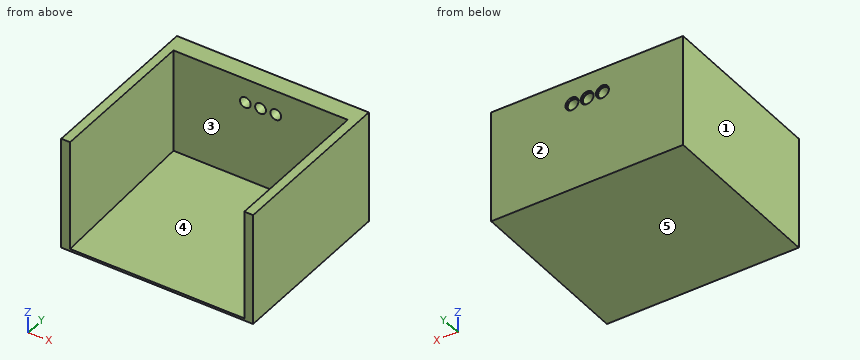
Autodesk Fusion 360 part; units mm, degrees
sketch "Sketch1" plane through (0, 0, 0) normal (0, 0, 1) x (1, 0, 0)
  line L0 (0, 0) -> (81, 0)
  line L1 (81, 0) -> (81, 71)
  line L2 (81, 71) -> (0, 71)
  line L3 (0, 71) -> (0, 0)
  dimension "d1" = 81
  dimension "d2" = 71
extrude "Extrude1" add sketch "Sketch1" along normal blind 1
sketch "Sketch2" plane through (0, 0, 0) normal (1, 0, 0) x (0, 1, 0)
sketch "Sketch3" plane through (0, 0, 1) normal (0, 0, 1) x (-1, 0, 0)
  line L0 (0, -71) -> (0, 0)
  line L1 (0, 0) -> (-81, 0)
  line L2 (-81, 0) -> (-81, -71)
  line L3 (-81, -71) -> (0, -71)
  line L4 (0, -71) -> (-1, -71)
  line L5 (-1, -71) -> (-1, 0)
  line L6 (-1, 0) -> (0, 0)
  line L7 (0, 0) -> (0, -71)
  line L8 (-81, -71) -> (-80, -71)
  line L9 (-80, -71) -> (-80, 0)
  line L10 (-80, 0) -> (-81, 0)
  line L11 (-81, 0) -> (-81, -71)
  line L12 (-1, -71) -> (-80, -71)
  line L13 (-80, -71) -> (-80, -70)
  line L14 (-80, -70) -> (-1, -70)
  line L15 (-1, -70) -> (-1, -71)
  dimension "d5" = 1
  dimension "d6" = 1
  dimension "d7" = 1
extrude "Extrude2" add sketch "Sketch3" along normal blind 50 contours L3 L5 L9 L12 L13 L14 L15
sketch "Sketch4" plane through (0, 0, 1) normal (0, 0, 1) x (-1, 0, 0)
  line L0 (-80, -71) -> (-80, -70)
  line L1 (-80, -70) -> (-1, -70)
  line L2 (-1, -70) -> (-1, -71)
  line L3 (-1, -71) -> (0, -71)
  line L4 (0, -71) -> (0, 0)
  line L5 (0, 0) -> (-81, 0)
  line L6 (-81, 0) -> (-81, -71)
  line L7 (-81, -71) -> (-80, -71)
  line L8 (0, 0) -> (-1, 0)
  line L9 (-1, 0) -> (-1, -71)
  line L10 (-1, -71) -> (0, -71)
  line L11 (0, -71) -> (0, 0)
  dimension "d10" = 1
  dimension "d11" = 71
extrude "Extrude3" add sketch "Sketch4" along normal blind 50 contours L2 L3 L4 L5 L8 L9 L10 L11
sketch "Sketch5" plane through (0, 0, 1) normal (0, 0, 1) x (-1, 0, 0)
  line L0 (-1, -70) -> (-1, 0)
  line L1 (-1, 0) -> (-81, 0)
  line L2 (-81, 0) -> (-81, -71)
  line L3 (-81, -71) -> (-80, -71)
  line L4 (-80, -71) -> (-80, -70)
  line L5 (-80, -70) -> (-1, -70)
  line L6 (-81, 0) -> (-80, 0)
  line L7 (-80, 0) -> (-80, -71)
  line L8 (-80, -71) -> (-81, -71)
  line L9 (-81, -71) -> (-81, 0)
  dimension "d14" = 71
extrude "Extrude4" add sketch "Sketch5" along normal blind 50 contours L1 L2 L3 L4 L6 L7 L8 L9
sketch "Sketch6" plane through (0, 70, 0) normal (0, -1, 0) x (1, 0, 0)
  line L0 (1, 1) -> (80, 1)
  line L1 (80, 1) -> (80, 51)
  line L2 (80, 51) -> (1, 51)
  line L3 (1, 51) -> (1, 1)
  line L4 (80, 1) -> (80, 4)
  line L5 (1, 4) -> (1, 1)
  dimension "d17" = 79
  dimension "d18" = 3
sketch "Sketch7" plane through (0, 70, 0) normal (0, -1, 0) x (1, 0, 0)
extrude "Extrude5" cut 1 faces at (27.3333, 46.6667, 1) along direction (0, 0, -1) blind 1
sketch "Sketch8" plane through (0, 0, 0) normal (0, 1, 0) x (1, 0, 0)
sketch "Sketch9" plane through (1, 0, 0) normal (1, 0, 0) x (0, 1, 0)
  line L0 (70, 0) -> (70, 51)
  line L1 (70, 51) -> (0, 51)
  line L2 (0, 51) -> (0, 0)
  line L3 (0, 0) -> (70, 0)
  line L4 (0, 0) -> (70, 0)
  line L5 (70, 0) -> (70, 1)
  line L6 (70, 1) -> (0, 1)
  line L7 (0, 1) -> (0, 0)
  dimension "d21" = 70
  dimension "d22" = 1
extrude "Extrude6" add sketch "Sketch9" along normal blind 79 contours L0 L2 L3 L4 L5 L6 L7
sketch "Sketch10" plane through (80, 0, 0) normal (-1, 0, 0) x (0, -1, 0)
  line L0 (-70, 1) -> (0, 1)
  line L1 (0, 1) -> (0, 51)
  line L2 (0, 51) -> (-70, 51)
  line L3 (-70, 51) -> (-70, 1)
  line L4 (-70, 1) -> (-70, 4)
  line L5 (-70, 4) -> (0, 1)
  line L6 (-70, 1) -> (-70, 4)
extrude "Extrude7" add sketch "Sketch10" along normal blind 79 contours L0 L3 L4 L5 L6
sketch "Sketch11" plane through (0, 0, 0) normal (0, 0, 1) x (1, 0, 0)
  line L0 (0, 0) -> (-3, 0)
  line L1 (-3, 0) -> (-3, 74)
  line L2 (-3, 74) -> (0, 74)
  line L3 (0, 74) -> (0, 0)
  dimension "d27" = 3
  dimension "d28" = 74
extrude "Extrude8" add sketch "Sketch11" along normal blind 51
sketch "Sketch12" plane through (0, 0, 0) normal (1, 0, 0) x (0, 1, 0)
  line L0 (71, 51) -> (71, 0)
  line L1 (71, 0) -> (74, 0)
  line L2 (74, 0) -> (74, 51)
  line L3 (74, 51) -> (71, 51)
  line L4 (74, 51) -> (71, 51)
  line L5 (71, 51) -> (71, 0)
  line L6 (71, 0) -> (74, 0)
  line L7 (74, 0) -> (74, 51)
extrude "Extrude9" add sketch "Sketch12" along normal blind 84
sketch "Sketch13" plane through (0, 71, 0) normal (0, -1, 0) x (1, 0, 0)
  line L0 (81, 51) -> (81, 0)
  line L1 (81, 0) -> (84, 0)
  line L2 (84, 0) -> (84, 51)
  line L3 (84, 51) -> (81, 51)
  line L4 (81, 51) -> (84, 51)
  line L5 (84, 51) -> (84, 0)
  line L6 (84, 0) -> (81, 0)
  line L7 (81, 0) -> (81, 51)
extrude "Extrude10" add sketch "Sketch13" along normal blind 71
sketch "Sketch14" plane through (0, 74, 0) normal (0, 1, 0) x (-1, 0, 0)
  line L0 (-84, 0) -> (3, 0)
  line L1 (3, 0) -> (3, 51)
  line L2 (3, 51) -> (-84, 51)
  line L3 (-84, 51) -> (-84, 0)
extrude "Extrude11" add sketch "Sketch14" along normal blind 4.3
sketch "Sketch15" plane through (0, 78.3, 0) normal (0, 1, 0) x (-1, 0, 0)
  line L0 (-84, 51) -> (-84, 0)
  line L1 (-84, 0) -> (3, 0)
  line L2 (3, 0) -> (3, 51)
  line L3 (3, 51) -> (-84, 51)
  line L4 (-79, 40) -> (-84, 40)
  circle A0 centre (-40.5, 40) radius 2.95
  dimension "d37" = 43.5
  dimension "d38" = 5.9
extrude "Extrude12" cut sketch "Sketch15" against normal blind 0.8 contours A0
sketch "Sketch16" plane through (0, 77.5, 0) normal (0, 1, 0) x (-1, 0, 0)
  circle A0 centre (-40.5, 40) radius 2.95
  circle A1 centre (-40.5, 40) radius 2.45
  dimension "d41" = 4.9
extrude "Extrude13" cut sketch "Sketch16" against normal blind 10 contours A1
sketch "Sketch17" plane through (0, 78.3, 0) normal (0, 1, 0) x (-1, 0, 0)
  circle A0 centre (-40.5, 40) radius 2.95
  line L0 (-84, 51) -> (-84, 0)
  line L1 (-84, 0) -> (3, 0)
  line L2 (3, 0) -> (3, 51)
  line L3 (3, 51) -> (-84, 51)
  line L4 (-40.5, 42.95) -> (-40.5, 40)
  line L5 (-40.5, 40) -> (-37.55, 40)
  line L6 (-37.55, 40) -> (-36.55, 40)
  line L7 (-36.55, 40) -> (-33.6, 40)
  circle A1 centre (-33.6, 40) radius 2.95
  dimension "d44" = 2.95
  dimension "d45" = 1
  dimension "d46" = 2.95
  dimension "d47" = 5.9
extrude "Extrude14" cut sketch "Sketch17" against normal blind 0.8 contours A1
sketch "Sketch18" plane through (0, 77.5, 0) normal (0, 1, 0) x (-1, 0, 0)
  circle A0 centre (-33.6, 40) radius 2.95
  circle A1 centre (-33.6, 40) radius 2.45
  dimension "d50" = 4.9
extrude "Extrude15" cut sketch "Sketch18" against normal blind 10 contours A1
sketch "Sketch19" plane through (0, 78.3, 0) normal (0, 1, 0) x (-1, 0, 0)
  circle A0 centre (-33.6, 40) radius 2.95
  circle A1 centre (-40.5, 40) radius 2.95
  line L0 (-84, 51) -> (-84, 0)
  line L1 (-84, 0) -> (3, 0)
  line L2 (3, 0) -> (3, 51)
  line L3 (3, 51) -> (-84, 51)
  line L4 (-40.5, 40) -> (-43.45, 40)
  line L5 (-43.45, 40) -> (-44.45, 40)
  line L6 (-44.45, 40) -> (-47.4, 40)
  circle A2 centre (-47.4, 40) radius 2.95
  dimension "d53" = 2.95
  dimension "d54" = 1
  dimension "d55" = 2.95
  dimension "d57" = 5.9
extrude "Extrude16" cut sketch "Sketch19" against normal blind 0.8 contours A2
sketch "Sketch20" plane through (0, 77.5, 0) normal (0, 1, 0) x (-1, 0, 0)
  circle A0 centre (-47.4, 40) radius 2.95
  circle A1 centre (-47.4, 40) radius 2.45
  dimension "d60" = 4.9
extrude "Extrude17" cut sketch "Sketch20" against normal blind 10 contours A1
sketch "Sketch21" plane through (0, 78.3, 0) normal (0, 1, 0) x (-1, 0, 0)
  circle A0 centre (-47.4, 40) radius 2.95
  circle A1 centre (-33.6, 40) radius 2.95
  circle A2 centre (-40.5, 40) radius 2.95
  line L0 (-84, 51) -> (-84, 0)
  line L1 (-84, 0) -> (3, 0)
  line L2 (3, 0) -> (3, 51)
  line L3 (3, 51) -> (-84, 51)
equation "d37 = ( 87 / 2 ) * 1 mm"
equation "d44 = ( 5.9 / 2 ) * 1 mm"
equation "d46 = ( 5.9 / 2 ) * 1 mm"
equation "d53 = ( 5.9 / 2 ) * 1 mm"
equation "d55 = ( 5.9 / 2 ) * 1 mm"
Check sheet for the modelled part. Datum: model origin and axes. Units: mm. Face numbers are marked on the shaded views. A direction names the side the tool comes from. Round coordinates to 2 decimals unless told otherwise and drop trailing zeros. Order: outer loops, then holes, each group sorted by start corner. A loop starts at its lowest first (then second) coordinate and runs counter-clockwise, first axis right, second up.
(1) Access from +Z, -Z, +X, -X, +Y, -Y to the whole of each face (thin tool, end or side, straight path). Record for the marked faces 4 and 5.
(2) Cross-section at A-A, the plane x = 40.5. Enter the section's corners in (y, z), and give its area (3 significant figures).
(3) Cross-section at D-D, the plane z = 24. Enter the section's corners in (x, y).
(4) Draft check along X on the marked faces 1, 2 and 3. Enter one of: pulls with the +X half, pulls with the -X half, needs draft (parallel to the pull), parting line crosses it, or undercut.
(5) Cross-section at C-C, the plane y = 53. Enter the section's corners in (x, z).
(6) Scan lines: probe 1 along X at (y, z) = (4, 5); probe 2 along Y at (x, z) = (17.5, 8); probe 3 along Z at (x, y) = (47.4, 78). Record each from-to range of solid material in increasing order.
(7) Go/stop test with flat-tipped pins: P1, Ø3, axis at x = 39.5, z = 39, coming from the +Y side; P2, Ø2, axis at x = 18.5, y = 39.5, coming from the +Z side; P3, Ø6.5, axis at x = 33.6, z = 40, coming from the -Y side; P4, Ø4.5, axis at x = 40.5, z = 40, coming from the -Y side. Record where each tip stops, or that it passes through.
(8) Cross-section at B-B, the plane z = 40. State how many separate pieces and enclosed holes the cut face has, and give its area (3 significant figures).
Check sheet entries:
1. face 4: +Z, -Y
1. face 5: -Z, +X, -X, +Y, -Y
2. outline: (0, 0) - (78.3, 0) - (78.3, 37.05) - (77.5, 37.05) - (77.5, 37.55) - (70, 37.55) - (70, 4) - (0, 1) - close; (70, 42.45) - (77.5, 42.45) - (77.5, 42.95) - (78.3, 42.95) - (78.3, 51) - (70, 51) - close
2. area: 557 mm2
3. outline: (-3, 0) - (1, 0) - (1, 70) - (80, 70) - (80, 0) - (84, 0) - (84, 78.3) - (-3, 78.3) - close
4. face 1: pulls with the -X half
4. face 2: needs draft
4. face 3: undercut
5. outline: (-3, 0) - (84, 0) - (84, 51) - (80, 51) - (80, 3.27) - (1, 3.27) - (1, 51) - (-3, 51) - close
6. probe 1: x = -3 to 1, 80 to 84
6. probe 2: y = 70 to 78.3
6. probe 3: z = 0 to 37.05, 42.95 to 51
7. P1: stops at y = 77.5
7. P2: stops at z = 2.74
7. P3: stops at y = 70
7. P4: passes through
8. separate pieces: 4
8. enclosed holes: 0
8. area: 1,160 mm2
